```python
from build123d import *

# Parameters (mm, degrees)
SKETCH1_W                    = 12.7
SKETCH1_H                    = 53.086
BOSS_EXTRUDE1_DEPTH          = 3.175
CSK_FOR_M3_SFHCS1_AT_2_COUNT = 2
CSK_FOR_M3_SFHCS1_AT_2_PITCH = 40.386


with BuildPart() as part:
    # Sketch1 → Boss-Extrude1 (new body)
    with BuildSketch(Plane(origin=(0, 0, 0), x_dir=(1, 0, 0), z_dir=(0, 1, 0))):
        with Locations((6.35, 26.543)):
            Rectangle(SKETCH1_W, SKETCH1_H)
    extrude(amount=BOSS_EXTRUDE1_DEPTH)

    # Sketch2 → CSK for M3 SFHCS1 (revolve, cut)
    with BuildSketch(Plane(origin=(6.35, 3.175, -6.35), x_dir=(0, 0, 1), z_dir=(1, 0, 0))):
        Polygon((0, 0), (0, 3.175), (1.7, 3.175), (1.7, 1.66), (3.36, 0), align=None)
    csk_for_m3_sfhcs1 = revolve(axis=Axis((6.35, 9.525, -6.35), (0, -1, 0)), mode=Mode.SUBTRACT)

    # CSK for M3 SFHCS1 at 2: CSK for M3 SFHCS1 ×2
    with Locations(*[(0, 0, -i * CSK_FOR_M3_SFHCS1_AT_2_PITCH) for i in range(1, CSK_FOR_M3_SFHCS1_AT_2_COUNT)]):
        add(csk_for_m3_sfhcs1, mode=Mode.SUBTRACT)


solid = part.part
```
Geometry check sheet. Reference: the model listing, model coordinates, mm. Give positions to 0.01 mm unless a question says otherwise; leave off trailing zeros. Write each loop counter-clockwise with the first axis right and the second up, starting at its lowest first coordinate (ties: lowest second). Pieces come first, ordered by that corner, then holes.
1) Gauge pin test, flat ends, axial feed: pin 1 (4 mm diameter, centred on x = 6.35, z = -46.736, fed in from -Y); pin 2 (5.5 mm diameter, centred on x = 6.35, z = -6.35, fed in from +Y) (3 decimals). Record the tip position at first contact, or that the pin passes through.
2) Release check for a two-part mould opening along X. For faces 1 (the conical face through (7.45, 1.62, -48.17)), 2 (the flat face through (6, 0, -27)), 3 (the flat face through (12.7, 2, -26)), 4 (the cylindrical face through (4.917, 0.768, -5.436)) record: pulls with the +X half, pulls with the -X half, needs draft (parallel to the pull), parting line crosses it, or undercut.
3) Section check B-B, the plane x = 6.35. Record the boundary of the cut face in (y, z) (3 decimals), and give its area (3 significant figures).
4) Material ranges on L1, parallel to Z at x = 6.35, y = 1; L2, parallel to X at y = 0.6, z = -6.35; L3, parallel to Z at x = 9, y = 3, recorded low to high.
5) Section check C-C, the plane y = 0.65. Record the boundary of the cut face in (x, z), and give its area (3 significant figures).
6) Section check A-A, the plane z = -6.35. Record the boundary of the cut face in (x, y) (3 decimals).
Computed:
1. pin 1: stops at y = 0
1. pin 2: stops at y = 2.565
2. face 1: undercut
2. face 2: needs draft
2. face 3: pulls with the +X half
2. face 4: undercut
3. outline: (0, -53.086) - (3.175, -53.086) - (3.175, -50.096) - (1.515, -48.436) - (0, -48.436) - close; (0, -45.036) - (1.515, -45.036) - (3.175, -43.376) - (3.175, -9.71) - (1.515, -8.05) - (0, -8.05) - close; (0, -4.65) - (1.515, -4.65) - (3.175, -2.99) - (3.175, 0) - (0, 0) - close
3. area: 141 mm2
4. L1: z = -53.09 to -48.44, -45.04 to -8.05, -4.65 to 0
4. L2: x = 0 to 4.65, 8.05 to 12.7
4. L3: z = -53.09 to -48.5, -44.97 to -8.12, -4.58 to 0
5. outline: (0, -53.09) - (12.7, -53.09) - (12.7, 0) - (0, 0) - close; hole circle Ø3.4 at (6.35, -46.74); hole circle Ø3.4 at (6.35, -6.35)
5. area: 656 mm2
6. outline: (0, 0) - (4.65, 0) - (4.65, 1.515) - (2.99, 3.175) - (0, 3.175) - close; (8.05, 0) - (12.7, 0) - (12.7, 3.175) - (9.71, 3.175) - (8.05, 1.515) - close
